Source: three-view drawing plus pictorial views. Frame: mm from the lowest corner of the part. A direction names the side the tool comes from. Give positions to 0.01 mm unless a question says otherwise; leave off trailing zeros. Order: outer loops, then holes, each group sorted by start corner. A loop starts at its lowest first (then second) coordinate and runs counter-clockwise, first axis right, second up.
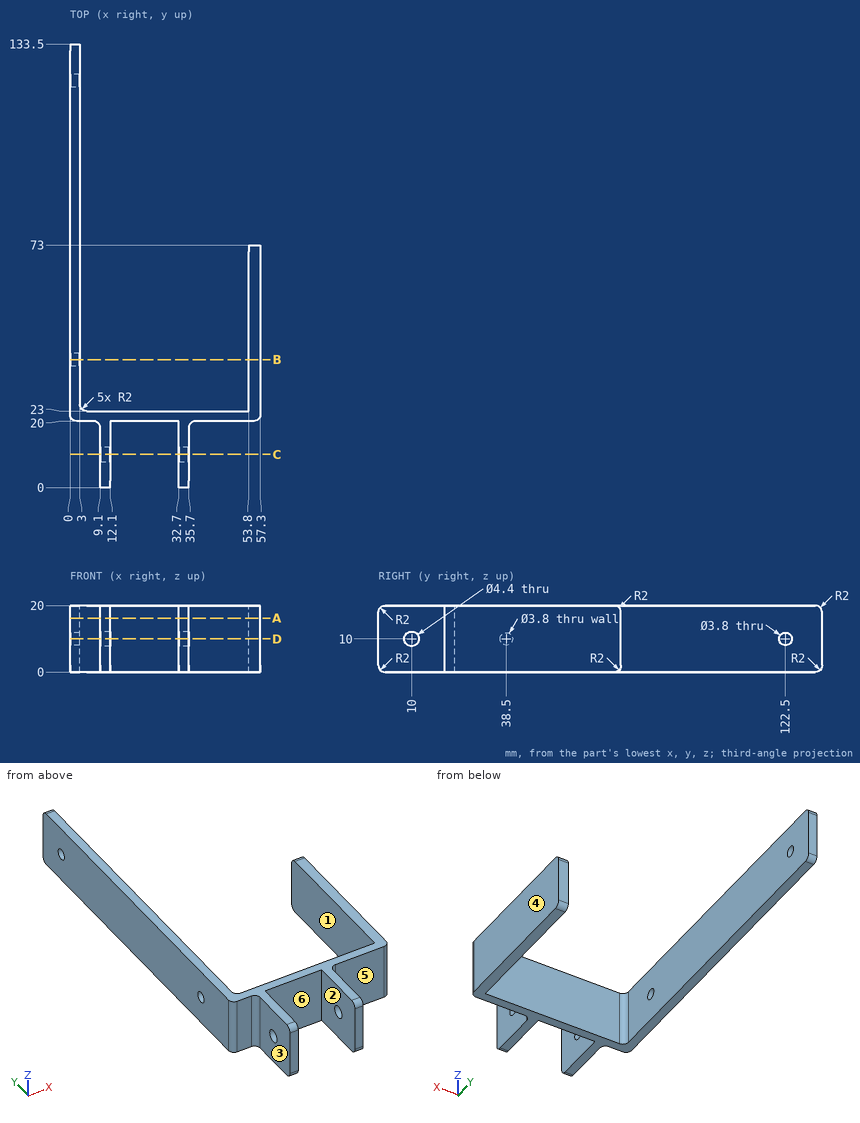
1) Section query A-A on z = 16.25. Output: boundary loops of the cut face in (x, y).
Checks:
outline: (0, 22) arc R2 ccw to (2, 20) - (7.1, 20) arc R2 cw to (9.1, 18) - (9.1, 0) - (12.1, 0) - (12.1, 20) - (32.7, 20) - (32.7, 0) - (35.7, 0) - (35.7, 18) arc R2 cw to (37.7, 20) - (55.3, 20) arc R2 ccw to (57.3, 22) - (57.3, 73) - (53.8, 73) - (53.8, 23) - (5, 23) arc R2 cw to (3, 25) - (3, 133.5) - (0, 133.5) - close
2) Section query B-B on y = 38.5. Output: boundary loops of the cut face in (x, z).
Checks:
outline: (0, 0) - (3, 0) - (3, 8.1) - (0, 8.1) - close; (0, 11.9) - (3, 11.9) - (3, 20) - (0, 20) - close; (53.8, 0) - (57.3, 0) - (57.3, 20) - (53.8, 20) - close
3) Section query D-D on z = 10. State how many separate pieces and enclosed holes the cut face has, and give its area (3 significant figures).
Checks:
separate pieces: 5
enclosed holes: 0
area: 750 mm2
4) Pull-direction query (X, two-part tool) for the marked faces 4, 5 and 6; classes: +X half, -X half, draft (parallel to the pull), parting line (faces both ways), or undercut.
Checks:
face 4: +X half
face 5: draft
face 6: undercut
5) Section query C-C on y = 10. Output: boundary loops of the cut face in (x, z), and give its area (3 significant figures).
Checks:
outline: (9.1, 0) - (12.1, 0) - (12.1, 7.8) - (9.1, 7.8) - close; (9.1, 12.2) - (12.1, 12.2) - (12.1, 20) - (9.1, 20) - close; (32.7, 0) - (35.7, 0) - (35.7, 7.8) - (32.7, 7.8) - close; (32.7, 12.2) - (35.7, 12.2) - (35.7, 20) - (32.7, 20) - close
area: 93.6 mm2
6) Ray query, L1, parallel to X at y = 69.5, z = 5.75; L2, parallel to X at y = 15, z = 19; L3, parallel to Z at x = 2.2, y = 122.5. Return the intervals inside material, ascending.
Checks:
L1: x = 0 to 3, 53.8 to 57.3
L2: x = 9.1 to 12.1, 32.7 to 35.7
L3: z = 0 to 8.1, 11.9 to 20
7) First-contact query: pin 1 Ø3.5 at (y, z) = (10, 10) entering from +X; pin 2 Ø5.5 at (y, z) = (10, 11.5) entering from +X; pin 3 Ø5 at (x, z) = (11.5, 8) entering from +Y; pin 4 Ø4 at (x, z) = (5.5, 13) entering from -Y. Flat tips, straight axial feed; report the tip coordinate or a pass-through.
Checks:
pin 1: passes through
pin 2: stops at x = 35.7
pin 3: stops at y = 23
pin 4: stops at y = 19.96
8) Reachability of the marked faces 1, 2 and 3 from +Z, -Z, +X, -X, +Y, -Y: full face, straight path, thin tool, end or side. Return the list, or none.
Checks:
face 1: +Z, -Z, +Y
face 2: +Z, -Z, -Y
face 3: +Z, -Z, -X, -Y
